Model file for the job. Use its own axes, mm. A direction names the side the tool comes from. Round coordinates to 2 decimals unless told otherwise and drop trailing zeros. Loops run counter-clockwise (first coordinate to the right, second up) from the corner with the lowest first, then second, coordinate; pieces in that order, holes last. Notation, with made-up numbers: (-0.75, 57.25) -> (15.25, 57.25) arc R21 ccw to (15.25, 89.25) -> close; hole circle Ø2 at (-0.75, 9.5). An arc over 180 degrees is marked (long way). Use a Markdown table: item, result.
from build123d import *

# Parameters (mm, degrees)
PAD_DEPTH    = 12
SKETCH001_R  = 1.75
POCKET_DEPTH = 5


with BuildPart() as part:
    # Sketch → Pad (new body)
    with BuildSketch(Plane.XZ):
        Polygon((-6.15, 0), (6.15, 0), (6.15, 2), (8.15, 2), (8.15, -2), (4.953939, -2), (4, -1.5), (-4, -1.5), (-4.953939, -2), (-8.15, -2), (-8.15, 2), (-6.15, 2), align=None)
    extrude(amount=PAD_DEPTH)

    # Sketch001 (on Face1 of Pad) → Pocket (cut)
    with BuildSketch(Plane(origin=(0, 0, 0), x_dir=(-1, 0, 0), z_dir=(0, 0, 1))):
        with Locations((0, 6)):
            Circle(SKETCH001_R)
    extrude(amount=-POCKET_DEPTH, mode=Mode.SUBTRACT)


solid = part.part
Q1. Drill centre lines: L1, parallel to X at y = -8.75, z = 1; L2, parallel to X at y = -6, z = -0.4; L3, parallel to Y at x = 0, z = -1. Where is each one in solid material? Low to high. Write a range as from..to.
Results list:
| item | result |
|---|---|
| L1 | x = -8.15..-6.15, 6.15..8.15 |
| L2 | x = -8.15..-1.75, 1.75..8.15 |
| L3 | y = -12..-7.75, -4.25..0 |
Q2. Band-saw the part on A-A, the plane x = 0. Give the cut face in (y, z), plus the area to 4 significant figures.
Results list:
| item | result |
|---|---|
| outline | (-12, -1.5) -> (-7.75, -1.5) -> (-7.75, 0) -> (-12, 0) -> close; (-4.25, -1.5) -> (0, -1.5) -> (0, 0) -> (-4.25, 0) -> close |
| area | 12.75 mm² |
Q3. Flat gauge pins, fed straight in: pin 1 (3 mm diameter, centred on x = 0, y = -6, fed in from -Z); pin 2 (2 mm diameter, centred on x = -2, y = -8, fed in from +Z); pin 3 (4 mm diameter, centred on x = -1.5, y = -6.5, fed in from -Z). Where does each tip first touch, or does it go through?
Results list:
| item | result |
|---|---|
| pin 1 | passes through |
| pin 2 | stops at z = 0 |
| pin 3 | stops at z = -1.5 |
Q4. Band-saw the part on D-D, the plane y = -1. Give the cut face in (x, z), plus the area to 3 significant figures.
Results list:
| item | result |
|---|---|
| outline | (-8.15, -2) -> (-4.95, -2) -> (-4, -1.5) -> (4, -1.5) -> (4.95, -2) -> (8.15, -2) -> (8.15, 2) -> (6.15, 2) -> (6.15, 0) -> (-6.15, 0) -> (-6.15, 2) -> (-8.15, 2) -> close |
| area | 36.1 mm² |
Q5. Pull direction Y, two halves, no side cores. Call faces 4 (the face through (6.15, -6, 1)), 5 (the face through (0.38, -4.29, -0.74)), 6 (the face through (0.1, -12, -0.4)): released by +Y, released by -Y, zero draft, split by the parting line, or undercut.
Results list:
| item | result |
|---|---|
| face 4 | zero draft |
| face 5 | undercut |
| face 6 | released by -Y |
Q6. Band-saw the part on B-B, the plane y = -6. Give the cut face in (x, z).
Results list:
| item | result |
|---|---|
| outline | (-8.15, -2) -> (-4.95, -2) -> (-4, -1.5) -> (-1.75, -1.5) -> (-1.75, 0) -> (-6.15, 0) -> (-6.15, 2) -> (-8.15, 2) -> close; (1.75, -1.5) -> (4, -1.5) -> (4.95, -2) -> (8.15, -2) -> (8.15, 2) -> (6.15, 2) -> (6.15, 0) -> (1.75, 0) -> close |
Q7. Band-saw the part on C-C, the plane z = -1. Give the cut face in (x, y).
Results list:
| item | result |
|---|---|
| outline | (-8.15, -12) -> (8.15, -12) -> (8.15, 0) -> (-8.15, 0) -> close; hole circle Ø3.5 at (0, -6) |
Q8. Tool access for faces 1 (the face through (-6.15, -6, 1)), 2 (the face through (-7, -6, -2)), 3 (the face through (2, -6, -1.5)): list every direction of +Z, -Z, +X, -X, +Y, -Y with a clear straight run to the whole face (end or side of a thin tool).
Results list:
| item | result |
|---|---|
| face 1 | +Z, +Y, -Y |
| face 2 | -Z, +X, -X, +Y, -Y |
| face 3 | -Z, +Y, -Y |
